```python
from build123d import *

# Parameters (mm, degrees)
BOSS_EXTRUDE1_DEPTH         = 18.25625
CUT_EXTRUDE1_DEPTH          = 590.645135899
F_1_4_CLEARANCE_HOLE1_D     = 6.7564
F_1_4_CLEARANCE_HOLE1_DEPTH = 18.25625
SKETCH5_W                   = 374.65
SKETCH5_H                   = 298.45
CUT_EXTRUDE2_DEPTH          = 590.645135899


with BuildPart() as part:
    # Sketch1 → Boss-Extrude1 (new body)
    with BuildSketch(Plane(origin=(0, 0, 0), x_dir=(1, 0, 0), z_dir=(0, 1, 0))):
        Polygon((-187.325, -558.8), (187.325, -558.8), (187.325, 0), (66.675, 0), (66.675, -107.95), (-66.675, -107.95), (-66.675, 0), (-187.325, 0), align=None)
    extrude(amount=BOSS_EXTRUDE1_DEPTH)

    # Sketch2 → Cut-Extrude1 (cut, through all)
    with BuildSketch(Plane(origin=(0, 18.25625, 0), x_dir=(1, 0, 0), z_dir=(0, 1, 0))):
        Polygon((-187.325, -201.6125), (-125.4125, -139.7), (-187.325, -77.7875), align=None)
        Polygon((125.4125, -139.7), (187.325, -201.6125), (187.325, -77.7875), align=None)
    extrude(amount=-CUT_EXTRUDE1_DEPTH, mode=Mode.SUBTRACT)

    # 1/4 Clearance Hole1
    with Locations(Plane(origin=(0, 18.25625, 0), x_dir=(1, 0, 0), z_dir=(0, 1, 0))):
        with Locations((-64.29375, -105.56875), (64.29375, -105.56875), (-128.785398023, -139.705301977), (128.785398023, -139.705301977)):
            Hole(F_1_4_CLEARANCE_HOLE1_D / 2, depth=F_1_4_CLEARANCE_HOLE1_DEPTH)

    # Sketch5 → Cut-Extrude2 (cut, through all)
    with BuildSketch(Plane(origin=(0, 18.25625, 0), x_dir=(1, 0, 0), z_dir=(0, 1, 0))):
        with Locations((0, -409.575)):
            Rectangle(SKETCH5_W, SKETCH5_H)
    extrude(amount=-CUT_EXTRUDE2_DEPTH, mode=Mode.SUBTRACT)


solid = part.part
```
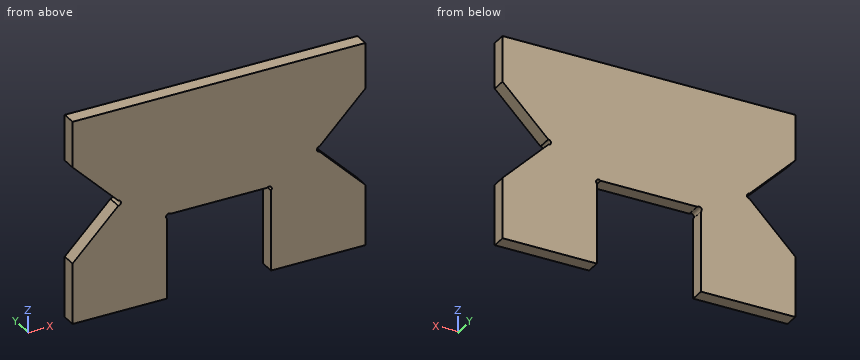
Model file for the job. Use its own axes, mm. Coordinates: 2 decimals unless noted, no trailing zeros. Loops run counter-clockwise (first coordinate to the right, second up) from the corner with the lowest first, then second, coordinate; pieces in that order, holes last. Notation, with made-up numbers: M -18.5,-17.75 L -12.5,-17.75 A13 ccw -12.5,0.25 Z; hole C 53,82.25 d9. An arc over 180 degrees is marked long. Use CSV: the item, a comma, the result in double quotes. Start each with the question number.
1. Band-saw the part on D-D, the plane x = 24. List the corners of the cut face in (y, z).
2. Band-saw the part on C-C, the plane x = -136. List the corners of the cut face in (y, z).
3. Flat gauge pins, fed straight in: pin 1 (2 mm diameter, centred on x = 42, y = 2.5, fed in from -Z); pin 2 (6 mm diameter, centred on y = 2, z = 152, fed in from -X); pin 3 (3 mm diameter, centred on y = 4, z = 199.5, fed in from +X). Where does each tip first touch, or does it go through?
4. Probe probe 1 along X at (y, z) = (8.75, 58.5) (3 decimals); probe 2 along Z at (x, y) = (33, 11); probe 3 along Z at (x, y) = (133.5, 6). List the from-to ranges inside material, lowest first. Write a range as [from, to].
5. Band-saw the part on A-A, the plane z = 22.5. List the corners of the cut face in (x, y) (3 decimals), then the cut area to 3 significant figures.
Entries:
1,outline,"M 0,107.95 L 18.26,107.95 L 18.26,260.35 L 0,260.35 Z"
2,outline,"M 0,0 L 18.26,0 L 18.26,129.11 L 0,129.11 Z; M 0,150.29 L 18.26,150.29 L 18.26,260.35 L 0,260.35 Z"
3,pin 1,"stops at z = 107.95"
3,pin 2,"stops at x = -140.71"
3,pin 3,"stops at x = 186.71"
4,probe 1,"x = [-187.325, -66.675], [66.675, 187.325]"
4,probe 2,"z = [107.95, 260.35]"
4,probe 3,"z = [0, 131.61], [147.79, 260.35]"
5,outline,"M -187.325,0 L -66.675,0 L -66.675,18.256 L -187.325,18.256 Z; M 66.675,0 L 187.325,0 L 187.325,18.256 L 66.675,18.256 Z"
5,area,"4,410 mm2"
